```python
from build123d import *

# Parameters (mm, degrees)
F1_DEPTH = 3


with BuildPart() as f1:
    # F0 (on Right) → F1 (new body)
    with BuildSketch(Plane.YZ):
        with BuildLine():
            Line((9, 34.019238), (0, 18.430781))
            Line((0, 18.430781), (0, 0))
            Line((0, 0), (70, 0))
            Line((70, 0), (70, 3))
            ThreePointArc((70, 3), (69.12132, 5.12132), (67, 6))
            Line((67, 6), (48.00438, 6))
            ThreePointArc((48.00438, 6), (45.875744, 6.475742), (44.152181, 7.812436))
            ThreePointArc((44.152181, 7.812436), (37.370731, 24.425762), (41.28461, 41.937822))
            Line((41.28461, 41.937822), (43.28461, 45.401924))
            ThreePointArc((43.28461, 45.401924), (43.584311, 47.678381), (42.186533, 49.5))
            Line((42.186533, 49.5), (24, 60))
            Line((24, 60), (15, 44.411543))
            Line((15, 44.411543), (12.401924, 45.911543))
            Line((12.401924, 45.911543), (6.401924, 35.519238))
            Line((6.401924, 35.519238), (9, 34.019238))
        make_face()
        Polygon((3.964102, 17.296806), (5.464102, 19.894882), (15.856406, 13.894882), (14.356406, 11.296806), align=None, mode=Mode.SUBTRACT)
        Polygon((26.320508, 24.019238), (32.320508, 34.411543), (34.918584, 32.911543), (28.918584, 22.519238), align=None, mode=Mode.SUBTRACT)
        Polygon((25.464102, 54.535898), (26.964102, 57.133975), (37.356406, 51.133975), (35.856406, 48.535898), align=None, mode=Mode.SUBTRACT)
    extrude(amount=F1_DEPTH)


solid = f1.part
```
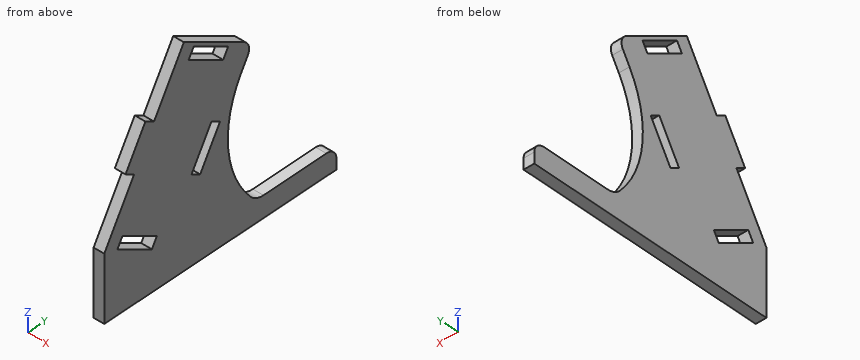
Can you work these out from the model? Positions are in its coordinate system, mm. Coordinates: 2 decimals unless noted, no trailing zeros. Order: outer loops, then holes, each group sorted by start corner. A loop starts at its lowest first (then second) coordinate and runs counter-clockwise, first axis right, second up. Notation, with made-up numbers: (-20, -32) -> (2, -32) arc R20 cw to (2, -1) -> close; hole circle Ø7 at (21.25, 0). An arc over 180 degrees is marked (long way). Write each question's results on one line, items separated by ' | '.
Item 1: I want a section at B-B, the plane z = 26. Write out the boundary of the cut face in (x, y).
Results are:
outline: (0, 4.37) -> (3, 4.37) -> (3, 27.46) -> (0, 27.46) -> close; (0, 30.93) -> (3, 30.93) -> (3, 37.28) -> (0, 37.28) -> close
Item 2: If I drill on line 1 along Z through (x, y) = (0.55, 52); line 2 along Z through (x, y) = (0.15, 40); line 3 along Z through (x, y) = (2.8, 29.5), over which ranges is the centre line in solid material (lowest first)?
Results are:
line 1: 0 to 6 | line 2: 0 to 14.42, 39.45 to 50.76 | line 3: 0 to 23.53, 29.53 to 52.21, 55.67 to 56.82
Item 3: I want a section at D-D, the plane z = 16. Write out the boundary of the cut face in (x, y), then the cut area to 4 significant figures.
Results are:
outline: (0, 0) -> (3, 0) -> (3, 6.21) -> (0, 6.21) -> close; (0, 12.21) -> (3, 12.21) -> (3, 39.33) -> (0, 39.33) -> close | area: 100.0 mm²
Item 4: I want a section at C-C, the plane y = 62.5. Write out the boundary of the cut face in (x, z), then the cut area to 3 significant figures.
Results are:
outline: (0, 0) -> (3, 0) -> (3, 6) -> (0, 6) -> close | area: 18.0 mm²
Item 5: I want a section at A-A, the plane x = 1.95. Write out the boundary of the cut face in (y, z).
Results are:
outline: (0, 0) -> (70, 0) -> (70, 3) arc R3 ccw to (67, 6) -> (48, 6) arc R5 cw to (44.15, 7.81) arc R30 cw to (41.28, 41.94) -> (43.28, 45.4) arc R3 ccw to (42.19, 49.5) -> (24, 60) -> (15, 44.41) -> (12.4, 45.91) -> (6.4, 35.52) -> (9, 34.02) -> (0, 18.43) -> close; hole (3.96, 17.3) -> (14.36, 11.3) -> (15.86, 13.89) -> (5.46, 19.89) -> close; hole (25.46, 54.54) -> (35.86, 48.54) -> (37.36, 51.13) -> (26.96, 57.13) -> close; hole (26.32, 24.02) -> (28.92, 22.52) -> (34.92, 32.91) -> (32.32, 34.41) -> close
Item 6: I'm going to push flat-ended pins straight in: pin 1 Ø1.5 at (x, y) = (1, 25) entering from +Z; pin 2 Ø1.5 at (x, y) = (1.5, 53.5) entering from +Z. Where does each tip first touch, or does it pass through?
Results are:
pin 1: z = 59.86 | pin 2: z = 6
